```python
from build123d import *

# Parameters (mm, degrees)
F1_DEPTH = 63.5
F2_DEPTH = 12.7
F0_W     = 50.3543876112
F0_H     = 10.7296556234
F0_W_2   = 5.8838576078
F0_H_2   = 6.9569721818


with BuildPart() as f1:
    # F0 (on Front) → F1 (new body, symmetric)
    with BuildSketch(Plane.XZ):
        Polygon((26.0407731761, 24.6988553554), (8.0104582012, 24.6988553554), (-36.4082939923, 24.6988553554), (-36.4082939923, -24.6988553554), (36.4082939923, -24.6988553554), (36.4082939923, 24.6988553554), align=None)
    extrude(amount=F1_DEPTH, both=True)

    # F0 (on Front) → F2 (join, symmetric)
    with BuildSketch(Plane.XZ):
        Polygon((45.6321343976, 66.9679120183), (8.0104582012, 24.6988553554), (26.0407731761, 24.6988553554), (63.6624493725, 66.9679120183), align=None)
    extrude(amount=F2_DEPTH, both=True)

    # F0 (on Front) → F3 (revolve)
    with BuildSketch(Plane.XZ):
        with Locations((109.4061043113, 72.33273983)):
            Rectangle(F0_W, F0_H)
        Polygon((78.3450528979, 72.33273983), (78.3450528979, 66.9679120183), (84.2289105058, 66.9679120183), (84.2289105058, 77.6975676417), (78.3450528979, 77.6975676417), align=None)
        with Locations((81.2869817019, 63.4894259274)):
            Rectangle(F0_W_2, F0_H_2)
        with Locations((81.2869817019, 81.1760537326)):
            Rectangle(F0_W_2, F0_H_2)
    revolve(axis=Axis((78.3450528979, 0, 78.4936398268), (0, 0, 1)))


solid = f1.part
```
Check sheet for the modelled part. Datum: model origin and axes. Units: mm. A direction names the side the tool comes from. Coordinates: 2 decimals unless noted, no trailing zeros. Write each loop counter-clockwise with the first axis right and the second up, starting at its lowest first coordinate (ties: lowest second). Pieces come first, ordered by that corner, then holes. Notation, with made-up numbers: M -36.75,59 L 5.25,59 A23 ccw 5.25,84 Z; hole C 53.25,8 d7. An arc over 180 degrees is marked long. Use one line per item in the form item = value.
Item 1: Sectioned sample at D-D, the plane z = 69.5. Record the cut outline in (x, y), and give its area (3 significant figures).
Answer below:
outline = C 78.35,0 d112.48
area = 9,940 mm^2
Item 2: Material ranges on L1, parallel to Z at x = -0.5, y = -26.5; L2, parallel to Z at x = 29, y = 13; L3, parallel to Z at x = 27.5, y = 1, recorded low to high. Write a range as from..to.
Answer below:
L1 = -24.7..24.7
L2 = -24.7..24.7, 66.97..77.7
L3 = -24.7..24.7, 26.34..46.6, 66.97..77.7
Item 3: Sectioned sample at B-B, the plane y = 0. Record the cut outline in (x, z), and give its area (3 significant figures).
Answer below:
outline = M -36.41,-24.7 L 36.41,-24.7 L 36.41,24.7 L 26.04,24.7 L 63.66,66.97 L 72.46,66.97 L 72.46,60.01 L 84.23,60.01 L 84.23,66.97 L 134.58,66.97 L 134.58,77.7 L 84.23,77.7 L 84.23,84.65 L 72.46,84.65 L 72.46,77.7 L 22.11,77.7 L 22.11,66.97 L 45.63,66.97 L 8.01,24.7 L -36.41,24.7 Z
area = 5,730 mm^2
Item 4: Release check for a two-part mould opening along Z. For faces 4 (the face through (36, 12.7, 44)), 5 (the face through (78, -12, 77.698)), 6 (the face through (83.78, -2.25, 63.54)) record: pulls with the +Z half, pulls with the -Z half, needs draft (parallel to the pull), parting line crosses it, or undercut.
Answer below:
face_4 = undercut
face_5 = pulls with the +Z half
face_6 = needs draft
Item 5: Sectioned sample at C-C, the plane y = -51. Record the cut outline in (x, z), and give its area (3 significant figures).
Answer below:
outline = M -36.41,-24.7 L 36.41,-24.7 L 36.41,24.7 L -36.41,24.7 Z; M 54.64,66.97 L 102.05,66.97 L 102.05,77.7 L 54.64,77.7 Z
area = 4,110 mm^2
Item 6: Set-up check for faces 1 (the face through (78, 0, 60.011)), 2 (the face through (36, -12.7, 44)), 3 (the face through (27.085, -0.178, 46.129)): record each of +Z, -Z, +X, -X, +Y, -Y from which the full face is reachable in a straight line by a thin tool's end or side.
Answer below:
face_1 = -Z, +X, +Y, -Y
face_2 = +X, -X, -Y
face_3 = -X, +Y, -Y
Item 7: Gauge pin test, flat ends, axial feed: pin 1 Ø6 at (x, y) = (108, -37) entering from +Z; pin 2 Ø4 at (y, z) = (-9.5, -2) entering from +X; pin 3 Ø21 at (x, z) = (30, 43.5) entering from +Y. Record the tip position at first contact, or that the pin passes through.
Answer below:
pin_1 = 77.7
pin_2 = 36.41
pin_3 = 12.7
Item 8: Sectioned sample at A-A, the plane x = 42. Record the cut outline in (y, z).
Answer below:
outline = M -42.92,66.97 L 42.92,66.97 L 42.92,77.7 L -42.92,77.7 Z; M -12.7,42.63 L 12.7,42.63 L 12.7,62.89 L -12.7,62.89 Z
